Design review of the part built by this model. Coordinates are the model's own, in mm. A direction names the side the tool comes from. Coordinates: 2 decimals unless noted, no trailing zeros. Loops run counter-clockwise (first coordinate to the right, second up) from the corner with the lowest first, then second, coordinate; pieces in that order, holes last. Notation, with made-up numbers: (59.25, 64.25) - (104.25, 64.25) arc R33 ccw to (104.25, 94.25) - close; hole circle Ø5 at (-3, -15.5). An arc over 180 degrees is marked (long way). Return JSON: item names as keys, results as strings. Group by question number.
from build123d import *

# Parameters (mm, degrees)
F0_R          = 18
F1_DEPTH      = 6
F1_DEPTH_BACK = 3
F1_TAPER_BACK = 30
F3_DEPTH      = 6.001
F5_D          = 11
F6_W          = 20
F6_H          = 5.5
F7_DEPTH      = 12.5
F8_R          = 2


with BuildPart() as f1:
    # F0 (on Top) → F1 (new body, two sides)
    with BuildSketch(Plane.XY) as f1_sk:
        Circle(F0_R)
    extrude(amount=F1_DEPTH)
    extrude(f1_sk.sketch, amount=-F1_DEPTH_BACK, taper=F1_TAPER_BACK)

    # F2 (on Top) → F3 (cut, through all)
    with BuildSketch(Plane.XY):
        with BuildLine():
            Line((-3.3431457505, 9), (-12.571075856, 14.3476765405))
            ThreePointArc((-12.571075856, 14.3476765405), (-14.1421356237, 14.1421356237), (-14.3476765405, 12.571075856))
            Line((-14.3476765405, 12.571075856), (-9, 3.3431457505))
            ThreePointArc((-9, 3.3431457505), (-7, 0), (-9, -3.3431457505))
            Line((-9, -3.3431457505), (-14.3476765405, -12.571075856))
            ThreePointArc((-14.3476765405, -12.571075856), (-14.1421356237, -14.1421356237), (-12.571075856, -14.3476765405))
            Line((-12.571075856, -14.3476765405), (-3.3431457505, -9))
            ThreePointArc((-3.3431457505, -9), (0, -7), (3.3431457505, -9))
            Line((3.3431457505, -9), (12.571075856, -14.3476765405))
            ThreePointArc((12.571075856, -14.3476765405), (14.1421356237, -14.1421356237), (14.3476765405, -12.571075856))
            Line((14.3476765405, -12.571075856), (9, -3.3431457505))
            ThreePointArc((9, -3.3431457505), (7, 0), (9, 3.3431457505))
            Line((9, 3.3431457505), (14.3476765405, 12.571075856))
            ThreePointArc((14.3476765405, 12.571075856), (14.1421356237, 14.1421356237), (12.571075856, 14.3476765405))
            Line((12.571075856, 14.3476765405), (3.3431457505, 9))
            ThreePointArc((3.3431457505, 9), (0, 7), (-3.3431457505, 9))
        make_face()
    extrude(amount=F3_DEPTH, mode=Mode.SUBTRACT)

    # F5 (through all)
    with Locations(Plane.XY):
        with Locations((0, 0)):
            Hole(F5_D / 2)

    # F6 (on Top) → F7 (cut, symmetric)
    with BuildSketch(Plane.XY):
        with Locations((-22, 0)):
            Rectangle(F6_W, F6_H)
        with Locations((22, 0)):
            Rectangle(F6_W, F6_H)
    extrude(amount=F7_DEPTH, both=True, mode=Mode.SUBTRACT)

    # F8
    f8_edges = [f1.edges().sort_by_distance(p)[0] for p in [
        (-12, 0, -3),
        (12, 0, -3),
    ]]
    fillet(f8_edges, radius=F8_R)


solid = f1.part
Item 1: Add section B-B (z = 2.5). State the section outline as (x, y) points.
Item 2: For faces 4 (the face through (6, 0, 0)), 5 (the face through (11.4, 0.04, -2.43)), 6 (the face through (12, 0, 3)), 7 (the face through (-12, 0, 2)), list the 3-axis set-ups (+Z, -Z, +X, -X, +Y, -Y) from which the entire face can be reached by the end or side of a thin tool; tool diameter is ignored.
Item 3: Add section A-A (y = 0). State the section outline as (x, z) points, then the cut area to 3 significant figures.
Item 4: Draft analysis for pull direction Y (two halves, no side actions). For faces 1 (the face through (-7, 0, 3)), 2 (the face through (7, 0, -3)), 3 (the face through (16.417, 7.38, 2.958)), state which applies: pulls with the +Y half, pulls with the -Y half, needs draft (parallel to the pull), parting line crosses it, or undercut.
Item 5: For P1, Ø4, axis at x = -13, z = 2, coming from the -Y side; P2, Ø3, axis at y = -0.5, z = 1, coming from the +X side; P3, Ø9, axis at x = 0, y = 0, coming from the -Z side; P4, Ø1, axis at x = -4.5, z = -1, coming from the +Y side, all flat-tipped, find the tip position at first contact; note any pin that passes through.
Item 6: To check wall thickness, follow line 1 (X direction, y = 9.5, z = 3.25); line 2 (Z direction, x = -10, y = 7.5); line 3 (X direction, y = -8, z = 1). State the ranges of each line that lie inside material, in increasing order. Write a range as from..to.
Item 7: Add section C-C (x = 0). State the section outline as (y, z) points.
Item 8: Add section D-D (z = -1.75). State the section outline as (x, y) points.
Answers below:
{
 "1": {"outline": "(-17.79, -2.75) arc R18 ccw to (-13.78, -11.59) - (-9, -3.34) arc R3.79 ccw to (-9, 3.34) - (-13.78, 11.59) arc R18 ccw to (-17.79, 2.75) - (-12, 2.75) - (-12, -2.75) - close; (-11.59, -13.78) arc R18 ccw to (11.59, -13.78) - (3.34, -9) arc R3.79 ccw to (-3.34, -9) - close; (-11.59, 13.78) - (-3.34, 9) arc R3.79 ccw to (3.34, 9) - (11.59, 13.78) arc R18 ccw to start; (9, -3.34) - (13.78, -11.59) arc R18 ccw to (17.79, -2.75) - (12, -2.75) - (12, 2.75) - (17.79, 2.75) arc R18 ccw to (13.78, 11.59) - (9, 3.34) arc R3.79 ccw to start"},
 "2": {"face 4": "+Z", "face 5": "-Z, +X", "face 6": "+Z, -Z, +X", "face 7": "+Z, -Z, -X"},
 "3": {"outline": "(-12, -1) arc R2 ccw to (-10, -3) - (-5.5, -3) - (-5.5, 0) - (-7, 0) - (-7, 6) - (-12, 6) - close; (5.5, -3) - (10, -3) arc R2 ccw to (12, -1) - (12, 6) - (7, 6) - (7, 0) - (5.5, 0) - close", "area": "97.3 mm^2"},
 "4": {"face 1": "undercut", "face 2": "needs draft", "face 3": "pulls with the +Y half"},
 "5": {"P1": "stops at y = -14.25", "P2": "stops at x = 12", "P3": "passes through", "P4": "stops at y = 17.16"},
 "6": {"line 1": "x = -15.29..-12.57, -4.21..4.21, 12.57..15.29", "line 2": "z = -3..0", "line 3": "x = -16.12..-11.7, -2.57..2.57, 11.7..16.12"},
 "7": {"outline": "(-18, 0) - (-16.27, -3) - (-5.5, -3) - (-5.5, 0) - (-7, 0) - (-7, 6) - (-18, 6) - close; (5.5, -3) - (16.27, -3) - (18, 0) - (18, 6) - (7, 6) - (7, 0) - (5.5, 0) - close"},
 "8": {"outline": "(-16.77, -2.75) arc R16.99 ccw to (16.77, -2.75) - (11.85, -2.75) - (11.85, 2.75) - (16.77, 2.75) arc R16.99 ccw to (-16.77, 2.75) - (-11.85, 2.75) - (-11.85, -2.75) - close; hole circle Ø11 at (0, 0)"}
}
